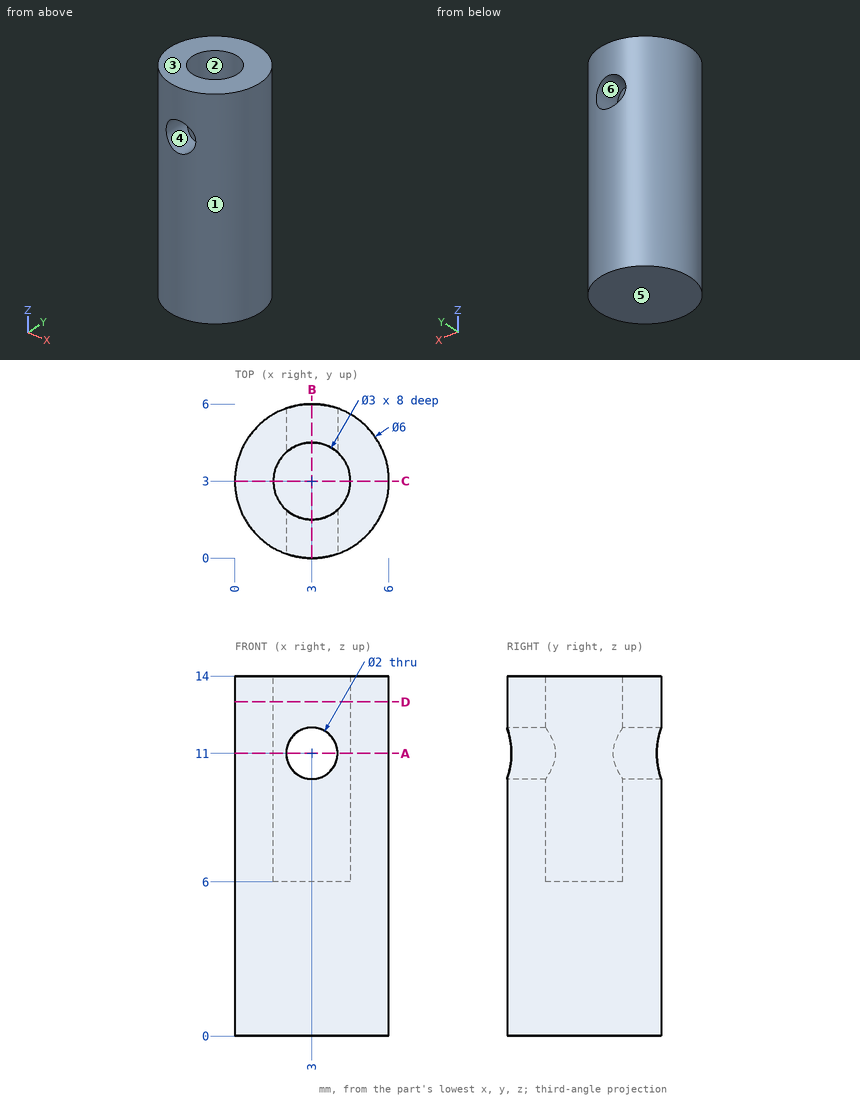
Part print with two shaded views. Sizes in mm from the minimum x, y, z corner. A direction names the side the tool comes from. Round coordinates to 2 decimals unless told otherwise and drop trailing zeros. Order: outer loops, then holes, each group sorted by start corner. A loop starts at its lowest first (then second) coordinate and runs counter-clockwise, first axis right, second up. Notation, with made-up numbers: M 63.25,-12.75 L 82.25,-12.75 A35 cw 82.25,21.25 Z; hole C 9.25,67.25 d4. An arc over 180 degrees is marked long. Use CSV: the item, a comma, the result in double quotes.
Item 1: Saw through at A-A (z = 11). List the corners of the cut face in (x, y).
Worked answers:
outline,"M 2,0.17 L 2,1.88 A1.5 cw 2,4.12 L 2,5.83 A3 ccw Z; M 4,0.17 A3 ccw 4,5.83 L 4,4.12 A1.5 cw 4,1.88 Z"
Item 2: Saw through at B-B (x = 3). List the corners of the cut face in (y, z), plus the area to 3 significant figures.
Worked answers:
outline,"M 0,0 L 6,0 L 6,10 L 4.5,10 L 4.5,6 L 1.5,6 L 1.5,10 L 0,10 Z; M 0,12 L 1.5,12 L 1.5,14 L 0,14 Z; M 4.5,12 L 6,12 L 6,14 L 4.5,14 Z"
area,"54.0 mm²"
Item 3: Which spindle directions (+Z, -Z, +X, -X, +Y, -Y) get a long thin tool onto all of the face, cutting with end or side? Do the marked faces 1 and 2. Say none if no direction does.
Worked answers:
face 1,"+Z, -Z"
face 2,"+Z"
Item 4: Saw through at D-D (z = 13). List the corners of the cut face in (x, y), plus the area to 3 significant figures.
Worked answers:
outline,"C 3,3 d6; hole C 3,3 d3"
area,"21.2 mm²"
Item 5: Pull direction Z, two halves, no side cores. Call the marked faces 3, 4, 5 and 6: released by +Z, released by -Z, zero draft, split by the parting line, or undercut.
Worked answers:
face 3,"released by +Z"
face 4,"undercut"
face 5,"released by -Z"
face 6,"undercut"
Item 6: Saw through at C-C (y = 3). List the corners of the cut face in (x, z).
Worked answers:
outline,"M 0,0 L 6,0 L 6,14 L 4.5,14 L 4.5,6 L 1.5,6 L 1.5,14 L 0,14 Z"
Item 7: Pin check, flat tips, straight feed: pin 1 (0.9 mm diameter, centred on x = 3.5, y = 2.5, fed in from +Z); pin 2 (2 mm diameter, centred on y = 5, z = 6, fed in from -X); pin 3 (1.6 mm diameter, centred on x = 3, z = 11, fed in from +Y). Stop position of each tip, or through.
Worked answers:
pin 1,"z = 6"
pin 2,"x = 0.17"
pin 3,"through"
Item 8: Probe probe 1 along Y at (x, z) = (3, 8.75); probe 2 along Z at (x, y) = (2.75, 2); probe 3 along X at (y, z) = (2.5, 8). List the from-to ranges inside material, lowest first.
Worked answers:
probe 1,"0 to 1.5, 4.5 to 6"
probe 2,"0 to 6"
probe 3,"0.04 to 1.59, 4.41 to 5.96"
